Source: CAD feature listing. Evaluate the final solid. Frame: model axes, mm. Coordinates: 2 decimals unless noted, no trailing zeros. Loops run counter-clockwise (first coordinate to the right, second up) from the corner with the lowest first, then second, coordinate; pieces in that order, holes last.
Autodesk Inventor part; units mm, degrees
ref_plane "YZ Plane" through (0, 0, 0) normal (1, 0, 0) x (0, 1, 0)
ref_plane "XZ Plane" through (0, 0, 0) normal (0, 1, 0) x (-1, 0, 0)
ref_plane "XY Plane" through (0, 0, 0) normal (0, 0, 1) x (1, 0, 0)
sketch "Sketch1" plane through (0, 0, 0) normal (0, 0, 1) x (1, 0, 0)
  line L0 (0, 68.58) -> (0, -11.43)
  line L1 (-151.8412, 0) -> (151.8412, 0)
  line L2 (108.458, 57.15) -> (-108.458, 57.15)
  line L3 (-108.458, 57.15) -> (-108.458, 0)
  line L4 (-108.458, 0) -> (108.458, 0)
  line L5 (108.458, 0) -> (108.458, 57.15)
  line L6 (-59.7, 12.7) -> (-92.7, 12.7) construction
  line L7 (-92.7, 12.7) -> (-92.7, 42.7) construction
  line L8 (-92.7, 42.7) -> (-59.7, 42.7) construction
  line L9 (-59.7, 42.7) -> (-59.7, 12.7) construction
  line L10 (-59.7, 12.7) -> (-92.7, 42.7) construction
  line L11 (-92.7, 12.7) -> (-59.7, 42.7) construction
  line L12 (11.884, 17.813) -> (36.884, 17.813) construction
  line L13 (36.884, 17.813) -> (36.884, 37.813) construction
  line L14 (36.884, 37.813) -> (11.884, 37.813) construction
  line L15 (11.884, 37.813) -> (11.884, 17.813) construction
  line L16 (11.884, 17.813) -> (36.884, 37.813) construction
  line L17 (36.884, 17.813) -> (11.884, 37.813) construction
  line L18 (101.6, 44.45) -> (-101.6, 44.45) construction
  line L19 (-101.6, 44.45) -> (-101.6, 12.7) construction
  line L20 (-101.6, 12.7) -> (101.6, 12.7) construction
  line L21 (101.6, 12.7) -> (101.6, 44.45) construction
  line L22 (101.6, 44.45) -> (-101.6, 12.7) construction
  line L23 (-101.6, 44.45) -> (101.6, 12.7) construction
  line L24 (-13.13, 17.018) -> (-35.13, 17.018) construction
  point P0 (0, 0)
  point P1 (101.6, 12.7)
  point P2 (-76.2, 27.7)
  point P3 (24.384, 27.813)
  point P4 (39.0271, 27.7128)
  point P5 (9.7409, 27.827)
  point P6 (-26.68, 49.53)
  point P7 (-52.08, 49.53)
  point P8 (0, 28.575)
  point P9 (-24.13, 17.018)
  dimension "d1" = 57.15
  dimension "d2" = 101.6
  dimension "d4" = 12.7
  dimension "d5" = 33
  dimension "d27" = 108.458
  dimension "d44" = 30
  dimension "d54" = 14.45
  dimension "d55" = 76.2
  dimension "d56" = 12.7
  dimension "d58" = 25
  dimension "d59" = 20
  dimension "d77" = 29.2862
  dimension "d78" = 14.6431
  dimension "d79" = 27.813
  dimension "d80" = 7.62
  dimension "d81" = 101.6
  dimension "d82" = 108.458
  dimension "d83" = 31.75
  dimension "d84" = 12.7
  dimension "d85" = 22
  dimension "d87" = 17.018
  dimension "d96" = 24.13
  dimension "d97" = 24.384
  dimension "d98" = 7.62
  dimension "d99" = 25.4
extrude "Extrusion1" add sketch "Sketch1" against normal blind 5.842
hole "Hole1" at (-101.6, 12.7, 0) at (101.6, 12.7, 0) at (-101.6, 44.45, 0) at (101.6, 44.45, 0) direction (0, 0, -1) diameter 5.461 end through all
sketch "Sketch3" plane through (0, 0, 0) normal (0, 0, 1) x (1, 0, 0)
  point P0 (0, 0)
hole "Hole4 Tap M3" at (-92.7, 42.7, 0) at (-59.7, 42.7, 0) at (-59.7, 12.7, 0) at (-92.7, 12.7, 0) at (-26.68, 49.53, 0) at (-52.08, 49.53, 0) direction (0, 0, -1) diameter 2.3622 end through all
fillet "Fillet2" radius 4.7498 4 edges at (-108.458, 57.15, -2.921) (108.458, 57.15, -2.921) (108.458, 0, -2.921) (-108.458, 0, -2.921)
hole "Hole5" at (36.884, 37.813, 0) at (36.884, 17.813, 0) at (11.884, 17.813, 0) at (11.884, 37.813, 0) at (39.0271, 27.7128, 0) at (9.7409, 27.827, 0) direction (0, 0, -1) diameter 2.3622 end through all
hole "Hole6" at (24.384, 27.813, 0) direction (0, 0, -1) diameter 22.86 end through all
hole "Hole7 Tap M4" at (-35.13, 17.018, 0) at (-13.13, 17.018, 0) direction (0, 0, -1) diameter 3.242 end through all
mirror "Mirror1" about plane through (0, 0, 0) normal (1, 0, 0) of "Hole4 Tap M3"
equation "\"d82\" = d27"
Q1. Draft query along X for faces 1 (the cylindrical face through (13.05, 29.3, -2.96)), 2 (the cylindrical face through (107.104, 1.428, -2.962)), 3 (the flat face through (-1, 0, -3)). Return one class per face: +X half, -X half, draft (parallel to the pull), parting line (faces both ways), or undercut.
Q2. Section B-B, the plane x = 31.5. Return the cut outline in (y, z).
Q3. Section C-C, the plane z = -3. Count the separate pieces of the cut face and the enclosed holes in it, plus the area to 3 significant figures.
Q4. Line query: line 1 along Y through (x, z) = (-59.7, -2); line 2 along Y through (x, z) = (-101.6, -2); line 3 along Y through (x, z) = (52.08, -3.3). Output: solid intervals per line, ascending.
Q5. Section A-A, the plane x = -101.6. Return the cut outline in (y, z).
Derived:
1. face 1: undercut
1. face 2: +X half
1. face 3: draft
2. outline: (0, -5.84) - (18.87, -5.84) - (18.87, 0) - (0, 0) - close; (36.76, -5.84) - (57.15, -5.84) - (57.15, 0) - (36.76, 0) - close
3. separate pieces: 1
3. enclosed holes: 25
3. area: 11,800 mm2
4. line 1: y = 0 to 11.52, 13.88 to 41.52, 43.88 to 57.15
4. line 2: y = 0 to 9.97, 15.43 to 41.72, 47.18 to 57.15
4. line 3: y = 0 to 48.35, 50.71 to 57.15
5. outline: (0, -5.84) - (9.97, -5.84) - (9.97, 0) - (0, 0) - close; (15.43, -5.84) - (41.72, -5.84) - (41.72, 0) - (15.43, 0) - close; (47.18, -5.84) - (57.15, -5.84) - (57.15, 0) - (47.18, 0) - close
